Could you check a few things on this model? Use its own coordinates, in mm. Face numbers are marked on the shaded views. A direction names the side the tool comes from. Round coordinates to 2 decimals unless told otherwise and drop trailing zeros. Write each loop counter-clockwise with the first axis right and the second up, starting at its lowest first coordinate (ties: lowest second). Pieces come first, ordered by that corner, then holes. Notation, with made-up numbers: (50, 43.25) -> (94, 43.25) arc R25 ccw to (94, 63.25) -> close; hole circle Ø2 at (75, 46.5). An arc over 180 degrees is marked (long way). Return JSON: item names as keys, results as strings.
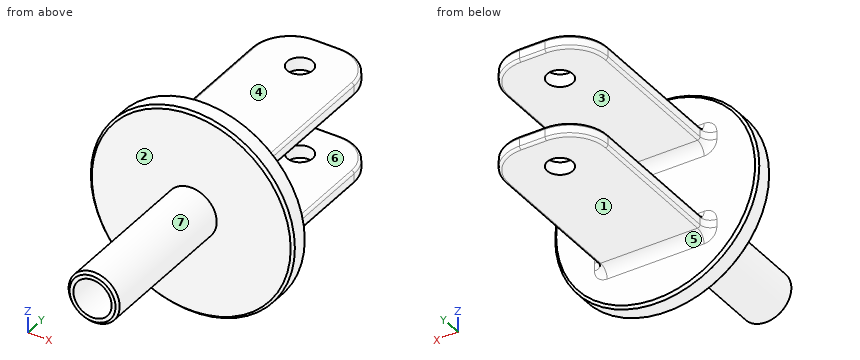
from build123d import *

# Parameters (mm, degrees)
SKETCH2_R            = 40
BOSS_EXTRUDE1_DEPTH  = 8
SKETCH6_R            = 10
SKETCH6_R_2          = 7.5
BOSS_EXTRUDE4_DEPTH  = 60
CHAMFER1_SIZE        = 1
SKETCH19_W           = 40
SKETCH19_H           = 5
BOSS_EXTRUDE5_DEPTH  = 75
FILLET1_R            = 15
FILLET2_R            = 1
FILLET3_R            = 4
FILLET1_OF_MIRROR2_R = 15
FILLET2_OF_MIRROR2_R = 1
FILLET3_OF_MIRROR2_R = 4
SKETCH21_R           = 5
CUT_EXTRUDE1_DEPTH   = 40


with BuildPart() as part:
    # Sketch2 → Boss-Extrude1 (new body)
    with BuildSketch(Plane(origin=(0, 0, 0), x_dir=(1, 0, 0), z_dir=(0, 1, 0))):
        Circle(SKETCH2_R)
    extrude(amount=BOSS_EXTRUDE1_DEPTH)

    # Sketch6 → Boss-Extrude4 (add)
    with BuildSketch(Plane.XZ):
        Circle(SKETCH6_R)
        Circle(SKETCH6_R_2, mode=Mode.SUBTRACT)
    extrude(amount=BOSS_EXTRUDE4_DEPTH)

    # Chamfer1
    chamfer1_edges = [part.edges().sort_by_distance(p)[0] for p in [
        (-40, 0, 0),
        (-40, 8, 0),
        (-10, -60, 0),
    ]]
    chamfer(chamfer1_edges, length=CHAMFER1_SIZE)

    # Sketch19 → Boss-Extrude5 (add)
    with BuildSketch(Plane(origin=(0, 8, 0), x_dir=(1, 0, 0), z_dir=(0, 1, 0))):
        with Locations((0, 17.5)):
            Rectangle(SKETCH19_W, SKETCH19_H)
    boss_extrude5 = extrude(amount=BOSS_EXTRUDE5_DEPTH)

    # Fillet1
    fillet1_edges = [part.edges().sort_by_distance(p)[0] for p in [
        (-20, 83, -17.5),
        (20, 83, -17.5),
    ]]
    fillet(fillet1_edges, radius=FILLET1_R)

    # Fillet2
    fillet2_edges = [part.edges().sort_by_distance(p)[0] for p in [
        (0, 83, -15),
        (0, 83, -20),
        (-20, 38, -20),
        (20, 38, -20),
        (-15.606601718, 78.606601718, -20),
        (15.606601718, 78.606601718, -20),
        (20, 38, -15),
        (-20, 38, -15),
        (-15.606601718, 78.606601718, -15),
        (15.606601718, 78.606601718, -15),
    ]]
    fillet(fillet2_edges, radius=FILLET2_R)

    # Fillet3
    fillet3_edges = [part.edges().sort_by_distance(p)[0] for p in [
        (0, 8, -20),
        (20, 8, -17.5),
        (0, 8, -15),
        (-20, 8, -17.5),
        (19.707106781, 8, -19.707106781),
        (19.707106781, 8, -15.292893219),
        (-19.707106781, 8, -19.707106781),
        (-19.707106781, 8, -15.292893219),
    ]]
    fillet(fillet3_edges, radius=FILLET3_R)

    # Mirror2: Boss-Extrude5 across plane
    add(boss_extrude5.mirror(Plane.XY))

    # Fillet1 of Mirror2
    fillet1_of_mirror2_edges = [part.edges().sort_by_distance(p)[0] for p in [
        (-20, 83, 17.5),
        (20, 83, 17.5),
    ]]
    fillet(fillet1_of_mirror2_edges, radius=FILLET1_OF_MIRROR2_R)

    # Fillet2 of Mirror2
    fillet2_of_mirror2_edges = [part.edges().sort_by_distance(p)[0] for p in [
        (0, 83, 15),
        (0, 83, 20),
        (-20, 38, 20),
        (20, 38, 20),
        (-15.606601718, 78.606601718, 20),
        (15.606601718, 78.606601718, 20),
        (20, 38, 15),
        (-20, 38, 15),
        (-15.606601718, 78.606601718, 15),
        (15.606601718, 78.606601718, 15),
    ]]
    fillet(fillet2_of_mirror2_edges, radius=FILLET2_OF_MIRROR2_R)

    # Fillet3 of Mirror2
    fillet3_of_mirror2_edges = [part.edges().sort_by_distance(p)[0] for p in [
        (0, 8, 20),
        (20, 8, 17.5),
        (0, 8, 15),
        (-20, 8, 17.5),
        (19.707106781, 8, 19.707106781),
        (19.707106781, 8, 15.292893219),
        (-19.707106781, 8, 19.707106781),
        (-19.707106781, 8, 15.292893219),
    ]]
    fillet(fillet3_of_mirror2_edges, radius=FILLET3_OF_MIRROR2_R)

    # Sketch21 → Cut-Extrude1 (cut)
    with BuildSketch(Plane.XY.offset(20)):
        with Locations((-0.54, 67)):
            Circle(SKETCH21_R)
    extrude(amount=-CUT_EXTRUDE1_DEPTH, mode=Mode.SUBTRACT)


solid = part.part
1) I want a section at C-C, the plane x = -0.54. Count the separate pieces of the cut face and the enclosed holes in it, and give its area (3 significant figures).
Return value:
{"separate pieces": "3", "enclosed holes": "0", "area": "1,600 mm²"}
2) I want a section at A-A, the plane y = 53.5. Please give me the cut outline in (x, z).
Return value:
{"outline": "(-20, -19) arc R1 ccw to (-19, -20) -> (19, -20) arc R1 ccw to (20, -19) -> (20, -16) arc R1 ccw to (19, -15) -> (-19, -15) arc R1 ccw to (-20, -16) -> close; (-20, 16) arc R1 ccw to (-19, 15) -> (19, 15) arc R1 ccw to (20, 16) -> (20, 19) arc R1 ccw to (19, 20) -> (-19, 20) arc R1 ccw to (-20, 19) -> close"}
3) I want a section at B-B, the plane z = 0. Please give me the cut outline in (x, y), and give its area (3 significant figures).
Return value:
{"outline": "(-40, 1) -> (-39, 0) -> (-10, 0) -> (-10, -59) -> (-9, -60) -> (-7.5, -60) -> (-7.5, 0) -> (7.5, 0) -> (7.5, -60) -> (9, -60) -> (10, -59) -> (10, 0) -> (39, 0) -> (40, 1) -> (40, 7) -> (39, 8) -> (-39, 8) -> (-40, 7) -> close", "area": "937 mm²"}
4) For the marked faces 1, 2 and 3, which set-ups out of +Z, -Z, +X, -X, +Y, -Y let a thin tool reach every point of the face, with its end or its side?
Return value:
{"face 1": "-Z, +X, -X, +Y", "face 2": "-Y", "face 3": "+X, -X, +Y"}
5) If I drill on probe 1 along Y at (x, z) = (0, 17); probe 2 along Z at (x, y) = (14.5, 28); probe 3 along Y at (x, z) = (-18, 5), over which ranges is the centre line in solid material (lowest first)? Write a range as [from, to].
Return value:
{"probe 1": "[0, 62.03], [71.97, 83]", "probe 2": "[-20, -15], [15, 20]", "probe 3": "[0, 8]"}
6) Thinking about a two-plate mould opening in Z: for the marked faces 4, 5, 6 and 7, which applies, pulls with the +Z half, pulls with the -Z half, needs draft (parallel to the pull), parting line crosses it, or undercut?
Return value:
{"face 4": "pulls with the +Z half", "face 5": "pulls with the -Z half", "face 6": "undercut", "face 7": "parting line crosses it"}
7) I want a section at D-D, the plane y = -26. Please give me the cut outline in (x, z), and give its area (3 significant figures).
Return value:
{"outline": "circle Ø20 at (0, 0); hole circle Ø15 at (0, 0)", "area": "137 mm²"}
8) Will these pins go through, and if not, where does the flat tip stop? pin 1 Ø8 at (y, z) = (52.5, 25) entering from -X; pin 2 Ø6 at (x, z) = (25, -23) entering from -Y; pin 3 Ø4 at (y, z) = (-0.5, 27.5) entering from +X; pin 4 Ø4 at (y, z) = (2.5, -13) entering from -X.
Return value:
{"pin 1": "through", "pin 2": "y = 0", "pin 3": "x = 30.24", "pin 4": "x = -38.46"}
